For this review, take the finished solid that the model builds, in its own axes (mm). A direction names the side the tool comes from. Round coordinates to 2 decimals unless told otherwise and drop trailing zeros. Loops run counter-clockwise (first coordinate to the right, second up) from the corner with the lowest first, then second, coordinate; pieces in that order, holes last. Notation, with made-up numbers: M -19,15.25 L 1,15.25 A19 ccw 1,23.25 Z; hole C 81,30 d8. An arc over 180 degrees is marked long. One line per question, with ' | ' between items. Start each with the question number.
1) For pin 1 Ø2.5 at (x, y) = (-7, 0.34) entering from +Z; pin 2 Ø2 at (y, z) = (1.5, 4) entering from -X; pin 3 Ø3 at (x, y) = (4.5, -3) entering from -Z; pin 4 Ø5 at (x, z) = (7, 5.5) entering from +Y, all flat-tipped, find the tip position at first contact; note any pin that passes through.
2) We need section D-D (y = 0). Give the boundary of the cut face in (x, z), and give its area (3 significant figures).
3) We need section A-A (z = 8.5). Give the boundary of the cut face in (x, y).
4) Mouldability with a two-part tool opening along Z and no side actions: class faces 3 (the face through (-19.43, -3.99, 11.4)), 4 (the face through (-17, -4, 10)), 5 (the face through (19.146, -0.676, 0.986)) as pulls with the +Z half, pulls with the -Z half, needs draft (parallel to the pull), parting line crosses it, or undercut.
5) We need section B-B (x = -17). Give the boundary of the cut face in (y, z), and give its area (3 significant figures).
6) For faces 1 (the face through (-0.3, -3, 5.8)), 2 (the face through (20, -4, 4)), list the 3-axis set-ups (+Z, -Z, +X, -X, +Y, -Y) from which the entire face can be reached by the end or side of a thin tool; tool diameter is ignored.
7) For probe 1 along X at (y, z) = (-3.25, 8.5); probe 2 along Z at (x, y) = (15, -3.25); probe 3 along Y at (x, z) = (-17, 1.1), list the stretches that pass through material, from the lowest coordinate up. Write a range as from..to.
8) We need section C-C (x = -13). Give the boundary of the cut face in (y, z), and give its area (3 significant figures).
Autodesk Inventor part; units mm, degrees
ref_plane "YZ Plane" through (0, 0, 0) normal (1, 0, 0) x (0, 1, 0)
ref_plane "XZ Plane" through (0, 0, 0) normal (0, 1, 0) x (-1, 0, 0)
ref_plane "XY Plane" through (0, 0, 0) normal (0, 0, 1) x (1, 0, 0)
sketch "Sketch1" plane through (0, 0, 0) normal (0, 0, 1) x (1, 0, 0)
  line L0 (-20, -3) -> (20, -3) construction
  circle A0 centre (-17, 0) radius 2.25
  circle A1 centre (17, 0) radius 2.25
  circle A2 centre (0, 0) radius 2.25
  circle A3 centre (-7, 0.3446) radius 1
  circle A4 centre (7, 0.3446) radius 1
  line L1 (-23.9554, 0) -> (25.6733, 0) construction
  line L2 (0, 11.421) -> (0, -11.2937) construction
  line L3 (-20, -3) -> (20, -3)
  line L4 (20, -3) -> (20, 3)
  line L5 (20, 3) -> (-20, 3)
  line L6 (-20, 3) -> (-20, -3)
  circle A5 centre (-11.8345, 1.6861) radius 0.5
  line L7 (-20, -3) -> (20, -3)
  line L8 (20, -3) -> (20, -5)
  line L9 (20, -5) -> (-20, -5)
  line L10 (-20, -5) -> (-20, -3)
  point P0 (0, 0)
  point P1 (0, -3)
  point P2 (0, -3)
  point P3 (-2.8751, -5.808)
  point P4 (2.8751, -5.808)
  dimension "d0" = 40
  dimension "d1" = 4.5
  dimension "d2" = 4.5
  dimension "d3" = 3
  dimension "d4" = 4.5
  dimension "d5" = 3
  dimension "d6" = 3.3446
  dimension "d7" = 3.3446
  dimension "d8" = 3
  dimension "d9" = 17
  dimension "d10" = 17
  dimension "d11" = 3
  dimension "d12" = 3
  dimension "d13" = 3
  dimension "d14" = 3
  dimension "d16" = 1
  dimension "d20" = 2
extrude "Extrusion1" add sketch "Sketch1" along normal blind 2 contours L6 L5 L4 L3
extrude "Extrusion2" add sketch "Sketch1" along normal blind 12 contours L3 L8 L9 L10
sketch "Sketch2" plane through (-20, -3, 2) normal (0, 1, 0) x (1, 0, 0)
  line L0 (0, 0) -> (40, 0)
  line L1 (0, 0) -> (0, -10)
  line L2 (40, -10) -> (0, -10)
  line L3 (40, 0) -> (40, -10)
  circle A0 centre (5, -6.5) radius 2.5
  circle A1 centre (35, -6.5) radius 2.5
  line L4 (20, 0) -> (20, -10) construction
  line L5 (0, -6.5) -> (40, -6.5) construction
  circle A2 centre (20, -6.5) radius 2.5
  point P0 (20, 2)
  dimension "d24" = 5
  dimension "d25" = 5
  dimension "d26" = 15
  dimension "d27" = 15
  dimension "d28" = 3.5
  dimension "d29" = 5
extrude "Extrusion3" cut sketch "Sketch2" against normal blind 7 contours A0 | A1 | A2
fillet "Fillet2" radius 2 2 edges at (20, -4, 12) (-20, -4, 12)
fillet "Fillet3" radius 1 2 edges at (20, 3, 1) (-20, 3, 1)
properties part number "Bar"
Answers below:
1) pin 1: z = 2 | pin 2: through | pin 3: z = 0 | pin 4: y = -3
2) outline: M -20,0 L -19.25,0 L -19.25,2 L -20,2 Z; M -14.75,0 L -7.94,0 L -7.94,2 L -14.75,2 Z; M -6.06,0 L -2.25,0 L -2.25,2 L -6.06,2 Z; M 2.25,0 L 6.06,0 L 6.06,2 L 2.25,2 Z; M 7.94,0 L 14.75,0 L 14.75,2 L 7.94,2 Z; M 19.25,0 L 20,0 L 20,2 L 19.25,2 Z | area: 45.5 mm^2
3) outline: M -20,-5 L -17.5,-5 L -17.5,-3 L -20,-3 Z; M -12.5,-5 L -2.5,-5 L -2.5,-3 L -12.5,-3 Z; M 2.5,-5 L 12.5,-5 L 12.5,-3 L 2.5,-3 Z; M 17.5,-5 L 20,-5 L 20,-3 L 17.5,-3 Z
4) face 3: pulls with the +Z half | face 4: undercut | face 5: needs draft
5) outline: M -5,0 L -2.25,0 L -2.25,2 L -3,2 L -3,7 L -5,7 Z; M -5,10 L -3,10 L -3,12 L -5,12 Z; M 2.25,0 L 3,0 L 3,2 L 2.25,2 Z | area: 21.0 mm^2
6) face 1: +Z, +X, -X, +Y | face 2: +Z, -Z, +X, +Y, -Y
7) probe 1: -20..-17.5, -12.5..-2.5, 2.5..12.5, 17.5..20 | probe 2: 0..6, 11..12 | probe 3: -5..-2.25, 2.25..3
8) outline: M -5,0 L 3,0 L 3,2 L -3,2 L -3,7 L -5,7 Z; M -5,10 L -3,10 L -3,12 L -5,12 Z | area: 30.0 mm^2
